The figure shows three views and two pictorial views of one solid part (mm, origin at its lowest corner). Answer the questions. A direction names the side the tool comes from. Coordinates: 2 decimals unless noted, no trailing zeros. Write each loop counter-clockwise with the first axis right and the second up, starting at its lowest first coordinate (ties: lowest second). Pieces come first, ordered by that corner, then holes. Notation, with made-up numbers: M -21,16 L -2,16 A13 ccw -2,27 Z; hole C -12.5,8 d7. An arc over 180 degrees is marked long. Answer as CSV lines item,"result".
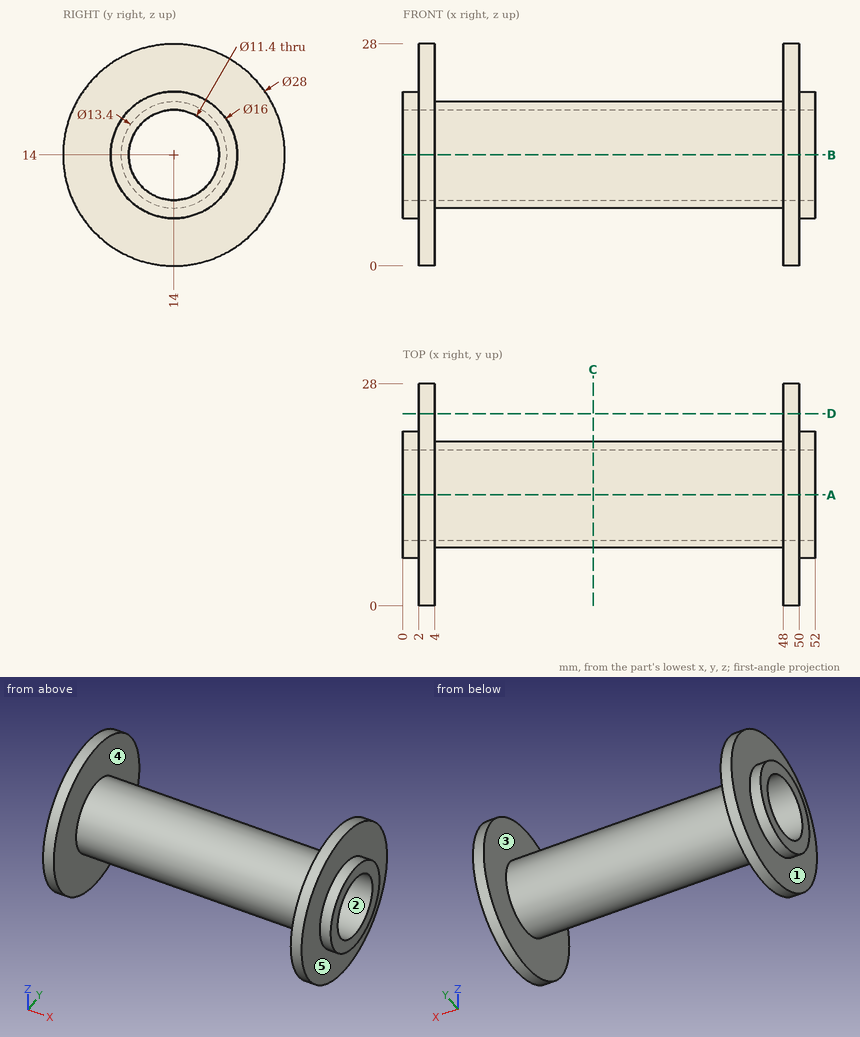
Q1. Find section C-C (x = 24). Give the vertices of the cut face in (y, z).
Output:
outline,"C 14,14 d13.4; hole C 14,14 d11.4"
Q2. Find section A-A (y = 14). Give the vertices of the cut face in (x, z).
Output:
outline,"M 0,6 L 2,6 L 2,0 L 4,0 L 4,7.3 L 48,7.3 L 48,0 L 50,0 L 50,6 L 52,6 L 52,8.3 L 0,8.3 Z; M 0,19.7 L 52,19.7 L 52,22 L 50,22 L 50,28 L 48,28 L 48,20.7 L 4,20.7 L 4,28 L 2,28 L 2,22 L 0,22 Z"
Q3. Find section D-D (y = 24.25). Give the vertices of the cut face in (x, z), and give its area (3 significant figures).
Output:
outline,"M 2,4.46 L 4,4.46 L 4,23.54 L 2,23.54 Z; M 48,4.46 L 50,4.46 L 50,23.54 L 48,23.54 Z"
area,"76.3 mm2"
Q4. For the marked faces 4 and 5, determine the directions among +Z, -Z, +X, -X, +Y, -Y from which every point of the face is accessible in a straight line to the end or side of a thin tool.
Output:
face 4,"none"
face 5,"+X"
Q5. Straight lines are drawn through the part: line 1 (Y direction, x = 15, z = 14); line 2 (X direction, y = 7.75, z = 25.25). For each, find the intervals that lie inside material, in ascending order.
Output:
line 1,"7.3 to 8.3, 19.7 to 20.7"
line 2,"2 to 4, 48 to 50"
Q6. Flat-ended cylindrical pins translate along their axes: pin 1 Ø2 at (x, y) = (19, 20.5) entering from -Z; pin 2 Ø5 at (x, z) = (26, 17.5) entering from -Y; pin 3 Ø5 at (x, y) = (14.5, 18.5) entering from +Z. Find the tip coordinate at first contact, or state that the pin passes through.
Output:
pin 1,"z = 10.17"
pin 2,"y = 7.38"
pin 3,"z = 20.39"
Q7. The mould has two halves that part along X. Classify the marked faces 1, 2 and 3: pulls with the +X half, pulls with the -X half, needs draft (parallel to the pull), parting line crosses it, or undercut.
Output:
face 1,"pulls with the -X half"
face 2,"needs draft"
face 3,"undercut"
